The model under review builds one solid part; all positions refer to its coordinate system, in mm. A direction names the side the tool comes from. Round coordinates to 2 decimals unless told otherwise and drop trailing zeros. Write each loop counter-clockwise with the first axis right and the second up, starting at its lowest first coordinate (ties: lowest second). Pieces come first, ordered by that corner, then holes. Notation, with made-up numbers: (69, -40) -> (89, -40) arc R16 ccw to (89, -32) -> close; hole circle Ø2 at (26, -36.75). An arc over 180 degrees is marked (long way). Answer in a Markdown table with one row per item. Add a question column.
```python
from build123d import *

# Parameters (mm, degrees)
BOSS_EXTRUDE1_DEPTH      = 20
BOSS_EXTRUDE1_DEPTH_BACK = 0.0001
SKETCH1_R                = 80
SKETCH2_R                = 60
BOSS_EXTRUDE2_DEPTH      = 40
SKETCH3_R                = 3
BOSS_EXTRUDE3_DEPTH      = 10
SKETCH4_R                = 2
CUT_EXTRUDE1_DEPTH       = 20
CHAMFER1_SIZE            = 20
SKETCH5_R                = 2


with BuildPart() as part:
    # Sketch1 → Boss-Extrude1 (new, two sides: drawn at the far end of the back side and taken through both)
    with BuildSketch(Plane(origin=(0, 0, 0), x_dir=(1, 0, 0), z_dir=(0, 1, 0)).offset(-BOSS_EXTRUDE1_DEPTH_BACK)):
        with Locations(Location((0, 0, 0), (0, 0, 270))):
            Circle(SKETCH1_R)
    extrude(amount=BOSS_EXTRUDE1_DEPTH + BOSS_EXTRUDE1_DEPTH_BACK)

    # Sketch2 → Boss-Extrude2 (add)
    with BuildSketch(Plane(origin=(0, 20, 0), x_dir=(1, 0, 0), z_dir=(0, 1, 0))):
        with Locations(Location((0, 0, 0), (0, 0, 270))):
            Circle(SKETCH2_R)
    extrude(amount=BOSS_EXTRUDE2_DEPTH)

    # Sketch3 → Boss-Extrude3 (add)
    with BuildSketch(Plane(origin=(0, 60, 0), x_dir=(1, 0, 0), z_dir=(0, 1, 0))):
        with Locations(Location((0, 0, 0), (0, 0, 270))):
            Circle(SKETCH3_R)
    extrude(amount=BOSS_EXTRUDE3_DEPTH)

    # Sketch4 → Cut-Extrude1 (cut)
    with BuildSketch(Plane(origin=(0, 70, 0), x_dir=(1, 0, 0), z_dir=(0, 1, 0))):
        with Locations(Location((0, 0, 0), (0, 0, 270))):
            Circle(SKETCH4_R)
    extrude(amount=-CUT_EXTRUDE1_DEPTH, mode=Mode.SUBTRACT)

    # Chamfer1
    chamfer1_edges = [part.edges().sort_by_distance(p)[0] for p in [
        (0, 20, -80),
    ]]
    chamfer(chamfer1_edges, length=CHAMFER1_SIZE - 0.0001)  # a hair under: the kernel refuses the full size

    # Sketch5 → Cut-Revolve1 (revolve, cut)
    with BuildSketch(Plane(origin=(0, 0, 0), x_dir=(0, 0, -1), z_dir=(1, 0, 0))):
        with Locations((-60, 56.839030786)):
            Circle(SKETCH5_R)
    revolve(axis=Axis((0, 60, 0), (0, -1, 0)), mode=Mode.SUBTRACT)

    # Fillet1: read off the stored shape, not the designer's step
    # Fillet1 outline → Fillet1 (revolve)
    with BuildSketch(Plane.XY):
        with BuildLine():
            ThreePointArc((62.928932188, 17.071067812), (60.761204675, 20.3153013), (60, 24.142135624))
            Line((60, 24.142135624), (60, 17.071067812))
            Line((60, 17.071067812), (62.928932188, 17.071067812))
        make_face()
    revolve(axis=Axis((0, 0, 0), (0, 1, 0)))


solid = part.part
```
1. Tool access review of faces 1 (the flat face through (-1, 70, 2)), 2 (the cylindrical face through (2.64, 59.41, -59.94)): name each direction out of +Z, -Z, +X, -X, +Y, -Y from which nothing blocks a thin tool from reaching the whole face with its end or side.
2. For L1, parallel to X at y = 63, z = 0; L2, parallel to Y at x = -47, z = 24.5; L3, parallel to X at y = 58, z = 0, list the stretches that pass through material, from the lowest coordinate up.
3. Insertion check: pin 1 Ø8 at (y, z) = (34, 23) entering from -X; pin 2 Ø8 at (x, y) = (24.5, 19.5) entering from -Z; pin 3 Ø2 at (y, z) = (9, -40.5) entering from +X; pin 4 Ø5 at (x, z) = (0, 0) entering from +Y. Each pin has a flat end and moves straight along its axis. Give the tip position at first contact, or say it passes through.
4. Mouldability with a two-part tool opening along X and no side actions: class faces 3 (the flat face through (1, 60, 12)), 4 (the cylindrical face through (0.9, 64.93, 2.86)), 5 (the flat face through (0, 50, 0)), 6 (the cylindrical face through (-2, 60, 0)) as pulls with the +X half, pulls with the -X half, needs draft (parallel to the pull), parting line crosses it, or undercut.
5. Add section C-C on y = 29. Write out the cut boundary in (x, z).
Filled in:
| question | item | result |
|---|---|---|
| 1 | face 1 | +Z, -Z, +X, -X, +Y |
| 1 | face 2 | +Y |
| 2 | L1 | -3 to -2, 2 to 3 |
| 2 | L2 | 0 to 60 |
| 2 | L3 | -58.37 to -2, 2 to 58.37 |
| 3 | pin 1 | x = -56.91 |
| 3 | pin 2 | z = -59.95 |
| 3 | pin 3 | x = 59.71 |
| 3 | pin 4 | y = 70 |
| 4 | face 3 | needs draft |
| 4 | face 4 | parting line crosses it |
| 4 | face 5 | undercut |
| 4 | face 6 | undercut |
| 5 | outline | circle Ø120 at (0, 0) |
